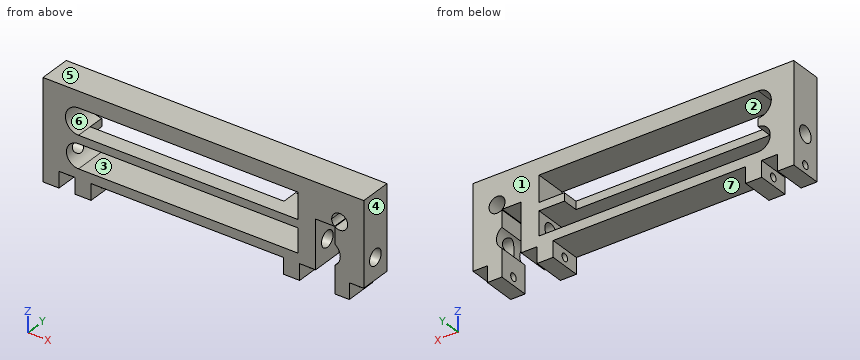
Autodesk Inventor part; units mm, degrees
ref_plane "YZ Plane" through (0, 0, 0) normal (1, 0, 0) x (0, 1, 0)
ref_plane "XZ Plane" through (0, 0, 0) normal (0, 1, 0) x (-1, 0, 0)
ref_plane "XY Plane" through (0, 0, 0) normal (0, 0, 1) x (1, 0, 0)
sketch "Sketch1" plane through (0, 0, 0) normal (0, 1, 0) x (-1, 0, 0)
  line L0 (31.75, -3.048) -> (-31.75, -3.048)
  line L1 (-31.75, -3.048) -> (-31.75, 0)
  line L2 (-31.75, 0) -> (31.75, 0)
  line L3 (31.75, 0) -> (31.75, -3.048)
  line L4 (-31.75, 0) -> (31.75, 0)
  line L5 (31.75, 0) -> (31.75, 16.5722)
  line L6 (31.75, 16.5722) -> (-31.75, 16.5722)
  line L7 (-31.75, 16.5722) -> (-31.75, 0)
  line L8 (24.7167, 10.8097) -> (-19.6375, 10.8097) construction
  line L9 (24.7167, 13.3972) -> (-19.6375, 13.3972)
  line L10 (-19.6375, 8.2222) -> (24.7167, 8.2222)
  arc A0 (24.7167, 8.2222) -> (24.7167, 13.3972) centre (24.7167, 10.8097) ccw
  arc A1 (-19.6375, 13.3972) -> (-19.6375, 8.2222) centre (-19.6375, 10.8097) ccw
  line L11 (24.7167, 4.2534) -> (-24.7167, 4.2534) construction
  line L12 (24.7167, 6.6347) -> (-24.7167, 6.6347)
  line L13 (-24.7167, 1.8722) -> (24.7167, 1.8722)
  arc A2 (24.7167, 1.8722) -> (24.7167, 6.6347) centre (24.7167, 4.2534) ccw
  arc A3 (-24.7167, 6.6347) -> (-24.7167, 1.8722) centre (-24.7167, 4.2534) ccw
  line L14 (0, 0) -> (0, 22.7513) construction
  circle A4 centre (-26.9875, 10.8097) radius 1.5875
  point P0 (0, 4.2534)
  dimension "d5" = 49.4334
  dimension "d6" = 5.175
  dimension "d7" = 4.7625
  dimension "d8" = 4.2534
  dimension "d23" = 7.0333
  dimension "d24" = 3.175
  dimension "d25" = 3.175
  dimension "d26" = 3.175
  dimension "d27" = 1.5875
  dimension "d28" = 3.175
extrude "Extrusion1" add sketch "Sketch1" along normal mid plane 6.35 contours L2 L7 L6 L5
sketch "Sketch3" plane through (0, 3.175, 0) normal (0, 1, 0) x (1, 0, 0)
  arc A0 (24.7167, -6.6347) -> (24.7167, -1.8722) centre (24.7167, -4.2534) ccw
  line L0 (24.7167, -4.2534) -> (4.7773, -4.2534) construction
  line L1 (26.045, -9.5942) -> (22.235, -9.5942)
  line L2 (22.235, -9.5942) -> (22.235, 1.0874)
  line L3 (22.235, 1.0874) -> (26.045, 1.0874)
  line L4 (26.045, 1.0874) -> (26.045, -9.5942)
  line L5 (26.045, -9.5942) -> (22.235, 1.0874) construction
  line L6 (22.235, -9.5942) -> (26.045, 1.0874) construction
  point P0 (0, 0)
  point P1 (24.14, -4.2534)
  dimension "d14" = 10.6816
  dimension "d15" = 3.81
extrude "Extrusion3" cut sketch "Sketch3" against normal through all contours L4 L1 L2 L3
sketch "Sketch4" plane through (0, 3.175, 0) normal (0, 1, 0) x (1, 0, 0)
  line L0 (22.235, -6.6347) -> (-24.7167, -6.6347)
  line L1 (22.235, -1.8722) -> (-24.7167, -1.8722)
  line L2 (22.235, -6.6347) -> (18.6822, -6.6347)
  line L3 (18.6822, -6.6347) -> (18.6822, -1.8722)
  line L4 (18.6822, -1.8722) -> (22.235, -1.8722)
  line L5 (22.235, -1.8722) -> (22.235, -6.6347)
  point P0 (0, 0)
  point P1 (22.235, -1.8722)
  point P2 (18.6822, -6.6347)
extrude "Extrusion4" add sketch "Sketch4" against normal up to surface (6.35 mm away)
sketch "Sketch2" plane through (31.75, -3.175, 0) normal (1, 0, 0) x (0, 0, -1)
  line L0 (0, 3.175) -> (-16.5722, 3.175) construction
  line L1 (-16.5722, 6.35) -> (-16.5722, 0) construction
  line L2 (-6.6347, 0) -> (-6.6347, 6.35) construction
  line L3 (-1.8722, 6.35) -> (-1.8722, 0) construction
  circle A0 centre (-4.2534, 3.175) radius 1.5875
  line L4 (-6.6347, 0) -> (-6.6347, 6.35) construction
  line L5 (-6.6347, -1.3931) -> (-4.2534, -1.3931) construction
  line L6 (-1.8722, 0) -> (-1.8722, 6.35) construction
  line L7 (-1.8722, -1.3931) -> (-4.2534, -1.3931) construction
  line L8 (-4.2534, -1.3931) -> (-4.2534, 6.8506) construction
  line L9 (-6.6347, 6.35) -> (-6.6347, 0)
  line L10 (-1.8722, 0) -> (-1.8722, 6.35)
  point P0 (-7.4284, 6.35)
  point P1 (-7.4284, 0)
  dimension "d9" = 3.175
extrude "Extrusion2" cut sketch "Sketch2" against normal through all
sketch "Sketch5" plane through (-24.7167, 3.175, 8.2222) normal (0, 0, 1) x (1, 0, 0)
  line L0 (24.7167, -3.175) -> (0, -3.175) construction
  line L1 (0, -6.35) -> (0, 0) construction
  line L2 (38.3736, -3.175) -> (0, -3.175)
  line L3 (0, -3.175) -> (0, 0)
  line L4 (0, 0) -> (38.3736, 0)
  line L5 (38.3736, 0) -> (38.3736, -3.175)
  line L6 (38.3736, -3.175) -> (0, 0) construction
  line L7 (0, -3.175) -> (38.3736, 0) construction
  line L8 (0, -6.35) -> (43.3989, -6.35)
  line L9 (43.3989, 0) -> (0, 0)
  point P0 (0, -3.175)
  dimension "d18" = 3.175
  dimension "d44" = 38.3736
extrude "Extrusion5" cut sketch "Sketch5" against normal up to next
sketch "Sketch6" plane through (31.75, -3.175, 0) normal (0, 0, -1) x (-1, 0, 0)
  line L0 (0, 7.366) -> (0, -4.826)
  line L1 (0, 6.35) -> (5.705, 6.35)
  line L2 (5.705, 0) -> (5.705, 6.35)
  line L3 (5.705, 0) -> (0, 0)
  line L4 (9.515, 6.35) -> (9.515, 0)
  line L5 (63.5, 0) -> (9.515, 0)
  line L6 (9.515, 0) -> (15.865, 0)
  line L7 (15.865, 0) -> (15.865, 6.35)
  line L8 (15.865, 6.35) -> (9.515, 6.35)
  line L9 (9.515, 6.35) -> (9.515, 0)
  line L10 (2.8525, 0) -> (2.8525, 6.35)
  line L11 (12.69, 0) -> (12.69, 6.35)
  line L12 (9.515, 6.35) -> (63.5, 6.35)
  line L13 (63.5, 0) -> (63.5, 6.35)
  line L14 (63.5, 0) -> (60.325, 0)
  line L15 (60.325, 0) -> (60.325, 6.35)
  line L16 (60.325, 6.35) -> (63.5, 6.35)
  line L17 (63.5, 6.35) -> (63.5, 0)
  line L18 (57.15, 0) -> (53.975, 0)
  line L19 (53.975, 0) -> (53.975, 6.35)
  line L20 (53.975, 6.35) -> (57.15, 6.35)
  line L21 (57.15, 6.35) -> (57.15, 0)
  point P0 (31.75, 3.175)
  point P1 (15.865, 0)
  point P2 (12.69, 0)
  dimension "d37" = 3.175
  dimension "d38" = 3.175
  dimension "d39" = 3.175
  dimension "d40" = 3.175
  dimension "d41" = 3.175
extrude "Extrusion6" add sketch "Sketch6" along normal blind 3.175 contours L1 L2 L3 L10 | L8 L7 L5 L11 | L12 L21 L5 L19 | L12 L13 L5 L15
sketch "Sketch7" plane through (31.75, -3.175, 16.5722) normal (1, 0, 0) x (0, 0, -1)
  circle A0 centre (18.1597, 3.175) radius 0.75
  line L0 (16.5722, 3.175) -> (19.7472, 3.175)
  line L1 (16.5722, 0) -> (0, 0)
  line L2 (0, 6.35) -> (16.5722, 6.35)
  line L3 (19.7472, 6.35) -> (19.7472, 0)
  dimension "d32" = 1.5
  dimension "d33" = 1.5875
extrude "Extrusion7" cut sketch "Sketch7" against normal through all
sketch "Sketch8" plane through (0, -3.175, 0) normal (0, -1, 0) x (1, 0, 0)
  line L0 (22.235, 0) -> (22.235, 9.5942)
  line L1 (22.235, 9.5942) -> (25.9663, 9.5942)
  arc A0 (26.045, 9.5323) -> (25.9663, 9.5942) centre (26.9875, 10.8097) ccw
  line L2 (26.045, 9.5323) -> (26.045, 6.2298)
  arc A1 (26.045, 2.277) -> (26.045, 6.2298) centre (24.7167, 4.2534) ccw
  line L3 (26.045, 2.277) -> (26.045, -3.175)
  line L4 (28.8975, -3.175) -> (26.045, -3.175)
  line L5 (28.8975, 0) -> (28.8975, -3.175)
  line L6 (28.8975, 0) -> (31.75, 0)
  line L7 (31.75, 0) -> (31.75, 16.5722)
  line L8 (31.75, 16.5722) -> (-31.75, 16.5722)
  line L9 (-31.75, 16.5722) -> (-31.75, -3.175)
  line L10 (-28.575, -3.175) -> (-31.75, -3.175)
  line L11 (-28.575, 0) -> (-28.575, -3.175)
  line L12 (-28.575, 0) -> (-25.4, 0)
  line L13 (-25.4, 0) -> (-25.4, -3.175)
  line L14 (-22.225, -3.175) -> (-25.4, -3.175)
  line L15 (-22.225, 0) -> (-22.225, -3.175)
  line L16 (-22.225, 0) -> (15.885, 0)
  line L17 (15.885, 0) -> (15.885, -3.175)
  line L18 (19.06, -3.175) -> (15.885, -3.175)
  line L19 (19.06, 0) -> (19.06, -3.175)
  line L20 (19.06, 0) -> (22.235, 0)
  line L21 (-24.7167, 13.3972) -> (19.6375, 13.3972)
  arc A2 (19.6375, 8.2222) -> (19.6375, 13.3972) centre (19.6375, 10.8097) ccw
  line L22 (19.6375, 8.2222) -> (-24.7167, 8.2222)
  arc A3 (-24.7167, 13.3972) -> (-24.7167, 8.2222) centre (-24.7167, 10.8097) ccw
  line L23 (18.6822, 6.6347) -> (18.6822, 1.8722)
  line L24 (18.6822, 1.8722) -> (-24.7167, 1.8722)
  arc A4 (-24.7167, 6.6347) -> (-24.7167, 1.8722) centre (-24.7167, 4.2534) ccw
  line L25 (-24.7167, 6.6347) -> (18.6822, 6.6347)
  line L26 (19.6375, 8.2222) -> (-24.7167, 8.2222)
  line L27 (18.6822, 8.2222) -> (18.6822, 13.3972)
  point P0 (0, 0)
extrude "Extrusion8" add sketch "Sketch8" against normal blind 6.35 contours L21 A2 L22 L27
properties part number "_3DPrint"
Work out the finished part from the listing and answer in its coordinate system (mm). Face numbers are marked on the shaded views. A direction names the side the tool comes from. Round coordinates to 2 decimals unless told otherwise and drop trailing zeros. Loops run counter-clockwise (first coordinate to the right, second up) from the corner with the lowest first, then second, coordinate; pieces in that order, holes last. Notation, with made-up numbers: (-14.75, 17.5) -> (12.25, 17.5) arc R22 cw to (12.25, 30.5) -> close; hole circle Ø11 at (34.5, 42.5). An arc over 180 degrees is marked (long way). Write each question's results on one line, items separated by ' | '. Start each with the question number.
1. For a pull along X with two mould halves and no side action, classify the marked faces 1, 2, 3 and 4 as +X half, -X half, draft (parallel to the pull), parting line (faces both ways), or undercut.
2. Section A-A (x = 4) is taken. Determine the outline of the cut face in (y, z) (3 decimals).
3. Find the intervals of material crossed by probe 1 along Z at (x, y) = (-1.5, -2); probe 2 along X at (y, z) = (1.5, 11); probe 3 along Z at (x, y) = (6.5, 2.5), in increasing order. Write a range as from..to.
4. Section B-B (z = 7.5) is taken. Determine the outline of the cut face in (x, y) (3 decimals), plus the area to 3 significant figures.
5. A tool of negligible diameter and unlimited length cuts with its end or side. For the marked faces 5, 6 and 7, from which of +Z, -Z, +X, -X, +Y, -Y can it reach the whole face along a straight path? Write none if from no direction.
6. Given pin 1 Ø3.5 at (y, z) = (-1, -2) entering from +X; pin 2 Ø1.9 at (x, y) = (-11, -0.5) entering from -Z, each flat-ended and moving along its own axis, determine where each tip first touches the part or whether it passes through.
Evaluation:
1) face 1: draft | face 2: undercut | face 3: undercut | face 4: +X half
2) outline: (-3.175, 0) -> (3.175, 0) -> (3.175, 1.872) -> (-3.175, 1.872) -> close; (-3.175, 6.635) -> (0, 6.635) -> (0, 8.222) -> (-3.175, 8.222) -> close; (-3.175, 13.397) -> (3.175, 13.397) -> (3.175, 16.572) -> (-3.175, 16.572) -> close
3) probe 1: z = 0..1.87, 6.63..8.22, 13.4..16.57 | probe 2: x = -31.75..-27.3, 18.68..25.41, 28.56..31.75 | probe 3: z = 0..1.87, 13.4..16.57
4) outline: (-31.75, -3.175) -> (22.235, -3.175) -> (22.235, 3.175) -> (13.657, 3.175) -> (13.657, 0) -> (-24.717, 0) -> (-24.717, 3.175) -> (-31.75, 3.175) -> close; (26.045, -3.175) -> (31.75, -3.175) -> (31.75, 3.175) -> (26.045, 3.175) -> close | area: 257 mm2
5) face 5: +Z, +X, -X, +Y, -Y | face 6: +Y, -Y | face 7: -Z, +Y, -Y
6) pin 1: stops at x = 28.9 | pin 2: stops at z = 0
